Check sheet for the modelled part. Datum: model origin and axes. Units: mm. A direction names the side the tool comes from. Round coordinates to 2 decimals unless told otherwise and drop trailing zeros. Order: outer loops, then holes, each group sorted by start corner. A loop starts at its lowest first (then second) coordinate and runs counter-clockwise, first axis right, second up. Notation, with made-up numbers: M 18,57 L 35,57 A10 ccw 35,76 Z; hole C 45,-26.75 d11. An arc over 180 degrees is marked long. One line per item, written item: value. Start each with the question number.
(1) Thickness scan on L1, parallel to Y at x = 0, z = 4.3; L2, parallel to X at y = 9.5, z = 5.15; L3, parallel to Y at x = 0, z = 1.5. Record the ranges inside material, lowest first.
(2) Release check for a two-part mould opening along X. For faces 1 (the face through (15.557, 27.683, 4.028)), 2 (the face through (22.5, 5, 3)), 3 (the face through (-13, 41, 6)) record: released by +X, released by -X, zero draft, split by the parting line, or undercut.
(3) Cross-section at B-B, the plane x = 3. Enter the section's corners in (y, z).
(4) Cross-section at C-C, the plane z = 4.25. Enter the section's corners in (x, y), and give its area (3 significant figures).
(5) Depth check by flat-ended pin: pin 1 Ø12 at (x, y) = (-7.5, 24.5) entering from -Z; pin 2 Ø2 at (x, z) = (-2, 5) entering from +Y; pin 3 Ø3 at (y, z) = (38.5, 3) entering from -X; pin 4 Ø6 at (x, y) = (0, 66) entering from +Z. Enter the tip coordinate at first touch or a pass-through.
(6) Cross-section at D-D, the plane y = 66. Enter the section's corners in (x, z), and give its area (3 significant figures).
(7) Cross-section at A-A, the plane z = 0.85. Enter the section's corners in (x, y).
(8) Access from +Z, -Z, +X, -X, +Y, -Y to the whole of each face (thin tool, end or side, straight path). Record for faces 4 (the face through (18.297, 4.141, 4.028)), 5 (the face through (16.223, 38.663, 2.958)).
Autodesk Inventor part; units mm, degrees
ref_plane "YZ Plane" through (0, 0, 0) normal (1, 0, 0) x (0, 1, 0)
ref_plane "XZ Plane" through (0, 0, 0) normal (0, 1, 0) x (-1, 0, 0)
ref_plane "XY Plane" through (0, 0, 0) normal (0, 0, 1) x (1, 0, 0)
sketch "Sketch1" plane through (0, 0, 0) normal (0, 0, 1) x (1, 0, 0)
  line L0 (-22.5, 0) -> (22.5, 0)
  line L1 (22.5, 0) -> (22.5, 10)
  line L2 (22.5, 10) -> (9.7685, 68.1391)
  arc A0 (9.7685, 68.1391) -> (-9.7685, 68.1391) centre (0, 66) ccw
  line L3 (-9.7685, 68.1391) -> (-22.5, 10)
  line L4 (-22.5, 10) -> (-22.5, 0)
  point P0 (0, 0)
  point P1 (0, 0)
  dimension "d0" = 45
  dimension "d1" = 10
  dimension "d2" = 10
  dimension "d3" = 66
extrude "Extrusion1" add sketch "Sketch1" along normal blind 6
sketch "Sketch2" plane through (0, 0, 6) normal (0, 0, 1) x (1, 0, 0)
  line L0 (22.5, 0) -> (22.5, 10)
  line L1 (22.5, 10) -> (9.7685, 68.1391)
  line L2 (-9.7685, 68.1391) -> (-22.5, 10)
  line L3 (-22.5, 10) -> (-22.5, 0)
  line L4 (-22.5, 0) -> (22.5, 0)
  line L5 (-19.5, 9.6754) -> (-11.7222, 45.1931)
  line L6 (11.7222, 45.1931) -> (19.5, 9.6754)
  line L7 (19.5, 9.6754) -> (19.5, 7)
  line L8 (15.5, 3) -> (-15.5, 3)
  line L9 (-19.5, 7) -> (-19.5, 9.6754)
  arc A0 (11.7222, 45.1931) -> (-11.7222, 45.1931) centre (0, 42.6261) ccw
  arc A1 (-19.5, 7) -> (-15.5, 3) centre (-15.5, 7) ccw
  arc A2 (15.5, 3) -> (19.5, 7) centre (15.5, 7) ccw
  point P0 (0, 0)
  dimension "d6" = 3
  dimension "d7" = 12
  dimension "d8" = 3
  dimension "d9" = 4
extrude "Extrusion2" cut sketch "Sketch2" against normal blind 4
sketch "Sketch3" plane through (0, 0, 6) normal (0, 0, 1) x (1, 0, 0)
  arc A0 (9.7685, 68.1391) -> (-9.7685, 68.1391) centre (0, 66) ccw
  point P0 (0, 0)
hole "Hole1" at (0, 66, 6) direction (0, 0, -1) diameter 10 end through all
properties part number "Bearing High" material "Steel"
Values found:
1. L1: 0 to 3, 54.63 to 61, 71 to 76
1. L2: -22.5 to -19.5, 19.5 to 22.5
1. L3: 0 to 61, 71 to 76
2. face 1: undercut
2. face 2: released by +X
2. face 3: zero draft
3. outline: M 0,0 L 62,0 L 62,6 L 54.25,6 L 54.25,2 L 3,2 L 3,6 L 0,6 Z; M 70,0 L 75.54,0 L 75.54,6 L 70,6 Z
4. outline: M -22.5,0 L 22.5,0 L 22.5,10 L 9.77,68.14 A10 ccw -9.77,68.14 L -22.5,10 Z; hole M -19.5,7 A4 ccw -15.5,3 L 15.5,3 A4 ccw 19.5,7 L 19.5,9.68 L 11.72,45.19 A12 ccw -11.72,45.19 L -19.5,9.68 Z; hole C 0,66 d10
4. area: 835 mm^2
5. pin 1: z = 0
5. pin 2: y = 75.95
5. pin 3: x = -16.59
5. pin 4: through
6. outline: M -10.24,0 L -5,0 L -5,6 L -10.24,6 Z; M 5,0 L 10.24,0 L 10.24,6 L 5,6 Z
6. area: 62.8 mm^2
7. outline: M -22.5,0 L 22.5,0 L 22.5,10 L 9.77,68.14 A10 ccw -9.77,68.14 L -22.5,10 Z; hole C 0,66 d10
8. face 4: +Z
8. face 5: +Z, -Z, +X, +Y
